The figure shows three views and two pictorial views of one solid part (mm, origin at its lowest corner). Answer the questions. Round coordinates to 2 decimals unless told otherwise and drop trailing zeros. Write each loop counter-clockwise with the first axis right and the second up, starting at its lowest first coordinate (ties: lowest second). Pieces come first, ordered by that corner, then holes.
Item 1: Each of these flat-tipped pins is pushed along its axis until it touches: pin 1 (4 mm diameter, centred on x = 5.5, y = 5.5, fed in from +Z); pin 2 (3.5 mm diameter, centred on x = 16.5, z = 16.5, fed in from -Y); pin 3 (5 mm diameter, centred on y = 6, z = 19.5, fed in from +X); pin 4 (1 mm diameter, centred on y = 8.5, z = 11.5, fed in from -X). Where does it stop, or does it pass through?
Item 2: For a pull along X with two mould halves and no side action, classify the marked faces 1, 2, 3 and 4 as +X half, -X half, draft (parallel to the pull), parting line (faces both ways), or undercut.
Item 3: Find section B-B on x = 11. Give the vertices of the cut face in (y, z), then the cut area to 3 significant figures.
Item 4: Find section C-C on y = 8.5. Give the vertices of the cut face in (x, z).
Item 5: Find the intervals of material crossed by probe 1 along Z at (x, y) = (11, 9.25); probe 2 along X at (y, z) = (10.7, 16.5) (3 decimals); probe 3 along Y at (x, z) = (4, 17.5), in increasing order.
Item 6: Find section A-A on z = 11. Give the vertices of the cut face in (x, y).
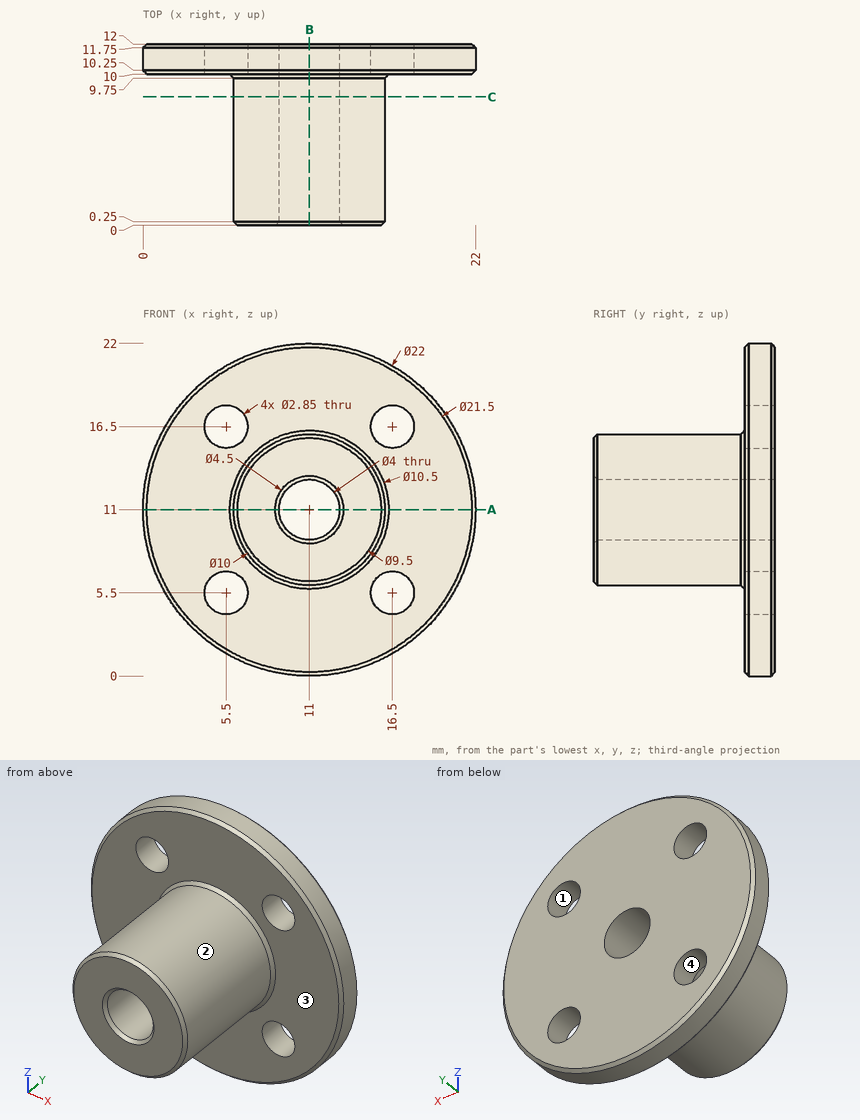
Check values:
1. pin 1: stops at z = 14.57
1. pin 2: stops at y = 10
1. pin 3: passes through
1. pin 4: stops at x = 6
2. face 1: undercut
2. face 2: parting line
2. face 3: draft
2. face 4: undercut
3. outline: (0, 6.25) - (0.25, 6) - (9.75, 6) - (10, 5.75) - (10, 0.25) - (10.25, 0) - (11.75, 0) - (12, 0.25) - (12, 9) - (0.25, 9) - (0, 8.75) - close; (0, 13.25) - (0.25, 13) - (12, 13) - (12, 21.75) - (11.75, 22) - (10.25, 22) - (10, 21.75) - (10, 16.25) - (9.75, 16) - (0.25, 16) - (0, 15.75) - close
3. area: 95.8 mm2
4. outline: circle Ø10 at (11, 11); hole circle Ø4 at (11, 11)
5. probe 1: z = 6 to 9, 13 to 16
5. probe 2: x = 1.474 to 4.075, 6.925 to 15.075, 17.925 to 20.526
5. probe 3: y = 10 to 12
6. outline: (0, 10.25) - (0.25, 10) - (5.75, 10) - (6, 9.75) - (6, 0.25) - (6.25, 0) - (8.75, 0) - (9, 0.25) - (9, 12) - (0.25, 12) - (0, 11.75) - close; (13, 0.25) - (13.25, 0) - (15.75, 0) - (16, 0.25) - (16, 9.75) - (16.25, 10) - (21.75, 10) - (22, 10.25) - (22, 11.75) - (21.75, 12) - (13, 12) - close
